Input: part model. Units: mm. Frame: model coordinates. A direction names the side the tool comes from. Coordinates: 2 decimals unless noted, no trailing zeros. Loops run counter-clockwise (first coordinate to the right, second up) from the corner with the lowest first, then second, coordinate; pieces in that order, holes last. Notation, with made-up numbers: (50, 43) -> (99, 43) arc R25 ccw to (99, 56) -> close; hole circle Ø2 at (15, -2). An arc over 180 degrees is marked (long way). Put each result on its own line as item: value. Start each with the question number.
1) Cut plane A-A (y = -8.5). Return the cut outline in (x, z).
2) Cut plane B-B (x = 31). Return the cut outline in (y, z), plus the area to 3 significant figures.
3) Contact query for flat-ended pins moving along their axis: P1, Ø12, axis at y = -2.5, z = 33.5, coming from the -X side; P2, Ø20.5, axis at y = 5, z = 22, coming from the +X side; P3, Ø14.5, axis at y = 1.5, z = 25.5, coming from the +X side. Output: stop coordinate, or through.
4) Material intervals for L1, parallel to X at y = 14.5, z = 32; L2, parallel to X at y = 20.5, z = 31; L3, parallel to Y at x = -28, z = 20, sorted ascending.
5) Set-up query: faces 4 (the flat face through (-16.857, 0, 25)), 5 (the cylindrical face through (44.252, 16.507, 25.044)), 6 (the flat face through (1, 29.971, 25)), 7 (the flat face through (-50, -17.271, 25)). Return all of +Z, -Z, +X, -X, +Y, -Y with unobstructed straight access to the full face (end or side cutting, diameter ignored); none if empty.
6) Pull-direction query (X, two-part tool) for faces 1 (the flat face through (53.687, -24, 25)), 2 (the cylindrical face through (17.621, -22.136, 25.044)), 3 (the flat face through (11, 0, 0)); classes: pulls with the +X half, pulls with the -X half, needs draft (parallel to the pull), parting line crosses it, or undercut.
7) Cut plane D-D (y = 16). Return the cut outline in (x, z).
8) Cut plane C-C (z = 7). State how many separate pieces and enclosed holes the cut face has, plus the area to 3 significant figures.
from build123d import *

# Parameters (mm, degrees)
F1_DEPTH = 50.8


with BuildPart() as f1:
    # F0 (on Top) → F1 (new body)
    with BuildSketch(Plane.XY):
        with BuildLine():
            Line((53.687494, 29.971173), (-53.687494, 29.971173))
            Line((-53.687494, 29.971173), (-53.687494, 17.271173))
            Line((-53.687494, 17.271173), (-46.067494, 17.271173))
            ThreePointArc((-46.067494, 17.271173), (-44.271443, 16.527224), (-43.527494, 14.731173))
            Line((-43.527494, 14.731173), (-43.527494, 0))
            Line((-43.527494, 0), (-34.637494, 0))
            Line((-34.637494, 0), (-34.637494, 20.32))
            ThreePointArc((-34.637494, 20.32), (-33.893545, 22.116051), (-32.097494, 22.86))
            Line((-32.097494, 22.86), (-19.397494, 22.86))
            ThreePointArc((-19.397494, 22.86), (-17.601443, 22.116051), (-16.857494, 20.32))
            Line((-16.857494, 20.32), (-16.857494, 0))
            Line((-16.857494, 0), (-8.89, 0))
            Line((-8.89, 0), (-8.89, 20.32))
            ThreePointArc((-8.89, 20.32), (-8.146051, 22.116051), (-6.35, 22.86))
            Line((-6.35, 22.86), (6.35, 22.86))
            ThreePointArc((6.35, 22.86), (8.146051, 22.116051), (8.89, 20.32))
            Line((8.89, 20.32), (8.89, 0))
            Line((8.89, 0), (16.857494, 0))
            Line((16.857494, 0), (16.857494, 20.32))
            ThreePointArc((16.857494, 20.32), (17.601443, 22.116051), (19.397494, 22.86))
            Line((19.397494, 22.86), (32.097494, 22.86))
            ThreePointArc((32.097494, 22.86), (33.893545, 22.116051), (34.637494, 20.32))
            Line((34.637494, 20.32), (34.637494, 0))
            Line((34.637494, 0), (43.527494, 0))
            Line((43.527494, 0), (43.527494, 14.731173))
            ThreePointArc((43.527494, 14.731173), (44.271443, 16.527224), (46.067494, 17.271173))
            Line((46.067494, 17.271173), (53.687494, 17.271173))
            Line((53.687494, 17.271173), (53.687494, 29.971173))
        make_face()
        with BuildLine():
            Line((-46.067494, -17.271173), (-53.687494, -17.271173))
            Line((-53.687494, -17.271173), (-53.687494, -29.971173))
            Line((-53.687494, -29.971173), (53.687494, -29.971173))
            Line((53.687494, -29.971173), (53.687494, -17.271173))
            Line((53.687494, -17.271173), (46.067494, -17.271173))
            ThreePointArc((46.067494, -17.271173), (44.271443, -16.527224), (43.527494, -14.731173))
            Line((43.527494, -14.731173), (43.527494, 0))
            Line((43.527494, 0), (34.637494, 0))
            Line((34.637494, 0), (34.637494, -20.32))
            ThreePointArc((34.637494, -20.32), (33.893545, -22.116051), (32.097494, -22.86))
            Line((32.097494, -22.86), (19.397494, -22.86))
            ThreePointArc((19.397494, -22.86), (17.601443, -22.116051), (16.857494, -20.32))
            Line((16.857494, -20.32), (16.857494, 0))
            Line((16.857494, 0), (8.89, 0))
            Line((8.89, 0), (8.89, -20.32))
            ThreePointArc((8.89, -20.32), (8.146051, -22.116051), (6.35, -22.86))
            Line((6.35, -22.86), (-6.35, -22.86))
            ThreePointArc((-6.35, -22.86), (-8.146051, -22.116051), (-8.89, -20.32))
            Line((-8.89, -20.32), (-8.89, 0))
            Line((-8.89, 0), (-16.857494, 0))
            Line((-16.857494, 0), (-16.857494, -20.32))
            ThreePointArc((-16.857494, -20.32), (-17.601443, -22.116051), (-19.397494, -22.86))
            Line((-19.397494, -22.86), (-32.097494, -22.86))
            ThreePointArc((-32.097494, -22.86), (-33.893545, -22.116051), (-34.637494, -20.32))
            Line((-34.637494, -20.32), (-34.637494, 0))
            Line((-34.637494, 0), (-43.527494, 0))
            Line((-43.527494, 0), (-43.527494, -14.731173))
            ThreePointArc((-43.527494, -14.731173), (-44.271443, -16.527224), (-46.067494, -17.271173))
        make_face()
    extrude(amount=F1_DEPTH)


solid = f1.part
Results found:
1. outline: (-43.53, 0) -> (-34.64, 0) -> (-34.64, 50.8) -> (-43.53, 50.8) -> close; (-16.86, 0) -> (-8.89, 0) -> (-8.89, 50.8) -> (-16.86, 50.8) -> close; (8.89, 0) -> (16.86, 0) -> (16.86, 50.8) -> (8.89, 50.8) -> close; (34.64, 0) -> (43.53, 0) -> (43.53, 50.8) -> (34.64, 50.8) -> close
2. outline: (-29.97, 0) -> (-22.86, 0) -> (-22.86, 50.8) -> (-29.97, 50.8) -> close; (22.86, 0) -> (29.97, 0) -> (29.97, 50.8) -> (22.86, 50.8) -> close
2. area: 722 mm2
3. P1: stops at x = -43.53
3. P2: stops at x = 43.58
3. P3: stops at x = 43.53
4. L1: x = -43.53 to -34.64, -16.86 to -8.89, 8.89 to 16.86, 34.64 to 43.53
4. L2: x = -53.69 to -34.63, -16.86 to -8.88, 8.88 to 16.86, 34.63 to 53.69
4. L3: y = -29.97 to -22.86, 22.86 to 29.97
5. face 4: +Z, -Z
5. face 5: +Z, -Z, +X
5. face 6: +Z, -Z, +X, -X, +Y
5. face 7: +Z, -Z, -X
6. face 1: pulls with the +X half
6. face 2: undercut
6. face 3: needs draft
7. outline: (-43.87, 0) -> (-34.64, 0) -> (-34.64, 50.8) -> (-43.87, 50.8) -> close; (-16.86, 0) -> (-8.89, 0) -> (-8.89, 50.8) -> (-16.86, 50.8) -> close; (8.89, 0) -> (16.86, 0) -> (16.86, 50.8) -> (8.89, 50.8) -> close; (34.64, 0) -> (43.87, 0) -> (43.87, 50.8) -> (34.64, 50.8) -> close
8. separate pieces: 1
8. enclosed holes: 3
8. area: 3,320 mm2
